from build123d import *

# Parameters (mm, degrees)
SKETCH1_W           = 42
SKETCH1_H           = 42
SKETCH1_R           = 1.9
BOSS_EXTRUDE1_DEPTH = 10
SKETCH2_W           = 12
SKETCH2_H           = 150
BOSS_EXTRUDE2_DEPTH = 10
SKETCH3_W           = 12
SKETCH3_H           = 3.75
BOSS_EXTRUDE3_DEPTH = 12
CHAMFER1_SIZE       = 3.75
CHAMFER1_SIZE_2     = 12.265697319
SKETCH4_R           = 1.375
CUT_EXTRUDE1_DEPTH  = 12
SKETCH5_W           = 42
SKETCH5_H           = 42
SKETCH5_R           = 1.65
SKETCH5_R_2         = 5
BOSS_EXTRUDE4_DEPTH = 7.5
SKETCH6_R           = 12.5
CUT_EXTRUDE2_DEPTH  = 5.2
FILLET1_R           = 4
FILLET2_R           = 9
SKETCH8_R           = 3.5
CUT_EXTRUDE4_DEPTH  = 1.2
BOSS_EXTRUDE7_DEPTH = 6


with BuildPart() as part:
    # Sketch1 → Boss-Extrude1 (new body)
    with BuildSketch(Plane(origin=(0, 0, 0), x_dir=(0, 0, -1), z_dir=(1, 0, 0))):
        Rectangle(SKETCH1_W, SKETCH1_H)
        with Locations((16, -16)):
            Circle(SKETCH1_R, mode=Mode.SUBTRACT)
        with Locations((-16, -16)):
            Circle(SKETCH1_R, mode=Mode.SUBTRACT)
        with Locations((-16, 16)):
            Circle(SKETCH1_R, mode=Mode.SUBTRACT)
        with Locations((16, 16)):
            Circle(SKETCH1_R, mode=Mode.SUBTRACT)
    extrude(amount=BOSS_EXTRUDE1_DEPTH)

    # Sketch2 → Boss-Extrude2 (add)
    with BuildSketch(Plane.ZY):
        with Locations((0, -29)):
            Rectangle(SKETCH2_W, SKETCH2_H)
    extrude(amount=-BOSS_EXTRUDE2_DEPTH)

    # Sketch3 → Boss-Extrude3 (add)
    with BuildSketch(Plane.ZY):
        with Locations((0, 40.375)):
            Rectangle(SKETCH3_W, SKETCH3_H)
        with Locations((0, -64.575)):
            Rectangle(SKETCH3_W, SKETCH3_H)
    extrude(amount=BOSS_EXTRUDE3_DEPTH)

    # Chamfer1
    # the kernel refuses this chamfer: 12.265697319, 3.75 mm, written as the material it adds along each edge
    with BuildSketch(Plane(origin=(0, 42.25, -6), x_dir=(0.11964200288050787, 0.9928170985366542, 0), z_dir=(0, 0, 1))) as chamfer1_piece_1_section:
        Polygon((CHAMFER1_SIZE * 0.992817098537, CHAMFER1_SIZE * 0.119642002881), (-CHAMFER1_SIZE_2 * 0.119642002884, CHAMFER1_SIZE_2 * 0.992817098562), (0, 0), align=None)
    chamfer1_piece_1 = extrude(amount=12, mode=Mode.PRIVATE)
    chamfer1_piece_1 = split(chamfer1_piece_1, bisect_by=Plane(origin=(-4.172539525, 46, 0), z_dir=(0, -1, 0)), keep=Keep.TOP, mode=Mode.PRIVATE)
    chamfer1_piece_1 = split(chamfer1_piece_1, bisect_by=Plane(origin=(-12, 43.383581674, 0), z_dir=(1, 0, 0)), keep=Keep.TOP, mode=Mode.PRIVATE)
    add(chamfer1_piece_1)
    with BuildSketch(Plane(origin=(0, -66.45, -6), x_dir=(0.11964200288050787, -0.9928170985366542, 0), z_dir=(0, 0, 1))) as chamfer1_piece_2_section:
        Polygon((CHAMFER1_SIZE * 0.992817098537, -CHAMFER1_SIZE * 0.119642002881), (-CHAMFER1_SIZE_2 * 0.119642002884, -CHAMFER1_SIZE_2 * 0.992817098562), (0, 0), align=None)
    chamfer1_piece_2 = extrude(amount=12, mode=Mode.PRIVATE)
    chamfer1_piece_2 = split(chamfer1_piece_2, bisect_by=Plane(origin=(-12, -67.58994207, 0), z_dir=(1, 0, 0)), keep=Keep.TOP, mode=Mode.PRIVATE)
    add(chamfer1_piece_2)

    # Sketch4 → Cut-Extrude1 (cut)
    with BuildSketch(Plane.ZY):
        with Locations((0, 25.4)):
            Circle(SKETCH4_R)
        with Locations((0, 0.4)):
            Circle(SKETCH4_R)
        with Locations((0, -24.6)):
            Circle(SKETCH4_R)
        with Locations((0, -49.6)):
            Circle(SKETCH4_R)
    extrude(amount=-CUT_EXTRUDE1_DEPTH, mode=Mode.SUBTRACT)

    # Sketch5 → Boss-Extrude4 (add)
    # profile 1 of 2: a face of its own
    with BuildSketch(Plane.XZ.offset(104)):
        Polygon((10, -56), (10, 6), (0, 6), (-34.5, -14), (7.5, -14), (7.5, -56), align=None)
    # profile 2 of 2: a face of its own
    with BuildSketch(Plane.XZ.offset(104)):
        with Locations((-13.5, -35)):
            Rectangle(SKETCH5_W, SKETCH5_H)
        with Locations(Location((-29, -50.5, 0), (0, 0, 270))):
            Circle(SKETCH5_R, mode=Mode.SUBTRACT)
        with Locations(Location((-13.5, -35, 0), (0, 0, 270))):
            Circle(SKETCH5_R_2, mode=Mode.SUBTRACT)
        with Locations(Location((2, -50.5, 0), (0, 0, 270))):
            Circle(SKETCH5_R, mode=Mode.SUBTRACT)
        with Locations(Location((-29, -19.5, 0), (0, 0, 270))):
            Circle(SKETCH5_R, mode=Mode.SUBTRACT)
        with Locations(Location((2, -19.5, 0), (0, 0, 270))):
            Circle(SKETCH5_R, mode=Mode.SUBTRACT)
    extrude(amount=BOSS_EXTRUDE4_DEPTH)

    # Sketch6 → Cut-Extrude2 (cut)
    with BuildSketch(Plane.XZ.offset(111.5)):
        with Locations(Location((-13.5, -35, 0), (0, 0, 270))):
            Circle(SKETCH6_R)
    extrude(amount=-CUT_EXTRUDE2_DEPTH, mode=Mode.SUBTRACT)

    # Fillet1
    fillet1_edges = [part.edges().sort_by_distance(p)[0] for p in [
        (-34.5, -107.75, -56),
        (10, -107.75, -56),
        (-34.5, -107.75, -14),
        (5, -21, 6),
        (5, -21, -6),
        (5, 21, -6),
        (5, 21, 6),
        (5, -21, -21),
        (5, -21, 21),
        (5, 21, 21),
        (5, 21, -21),
    ]]
    fillet(fillet1_edges, radius=FILLET1_R)

    # Fillet2
    fillet2_edges = [part.edges().sort_by_distance(p)[0] for p in [
        (5, -104, -6),
        (0, -104, 0),
    ]]
    fillet(fillet2_edges, radius=FILLET2_R)

    # Sketch8 → Cut-Extrude4 (cut)
    with BuildSketch(Plane(origin=(0, -104, 0), x_dir=(1, 0, 0), z_dir=(0, 1, 0))):
        with Locations(Location((-29, 50.5, 0), (0, 0, 270))):
            Circle(SKETCH8_R)
        with Locations(Location((2, 50.5, 0), (0, 0, 270))):
            Circle(SKETCH8_R)
        with Locations(Location((2, 19.5, 0), (0, 0, 270))):
            Circle(SKETCH8_R)
        with Locations(Location((-29, 19.5, 0), (0, 0, 270))):
            Circle(SKETCH8_R)
    extrude(amount=-CUT_EXTRUDE4_DEPTH, mode=Mode.SUBTRACT)

    # Sketch11 → Boss-Extrude7 (add)
    with BuildSketch(Plane.XZ.offset(111.5)):
        Polygon((8.3, 6), (10, 6), (10, 9.2), (2.9, 9.2), (2.9, 7.5), (3.9, 7.5), (8.3, 7.5), align=None)
        Polygon((3.9, 7.5), (2.9, 7.5), (3.433368825, 6.8), align=None)
    extrude(amount=-BOSS_EXTRUDE7_DEPTH)


solid = part.part
Work out the finished part from the listing and answer in its coordinate system (mm). A direction names the side the tool comes from. Give positions to 0.01 mm unless a question says otherwise; leave off trailing zeros. Order: outer loops, then holes, each group sorted by start corner. A loop starts at its lowest first (then second) coordinate and runs counter-clockwise, first axis right, second up. Notation, with made-up numbers: (-9.75, -16.75) -> (29.25, -16.75) arc R32 cw to (29.25, 21.25) -> close; hole circle Ø9 at (2.5, 21.5). An arc over 180 degrees is marked (long way). Answer as a JSON object with one key per item and string values. Group by question number.
1. The mould has two halves that part along X. Classify faces 5 (the flat face through (-6, 38.5, 0)), 6 (the cylindrical face through (-12.95, -108.936, -22.512)), 7 (the cylindrical face through (-33.98, -107.8, -14.33)), 8 (the flat face through (-31, -105.2, -19)): released by +X, released by -X, zero draft, split by the parting line, or undercut.
2. Section C-C on x = -13.5 is taken. Determine the outline of the cut face in (y, z).
3. Section D-D on z = -19.5 is taken. Determine the outline of the cut face in (x, y).
4. Consider line 1 along Y through (x, z) = (5.75, -16); line 2 along X through (y, z) = (-104.5, -19.5); line 3 along X through (y, z) = (-109, -50.5). Determine where each line is inside the solid, lowest interval first. Write a range as [from, to].
5. A tool of negligible diameter and unlimited length cuts with its end or side. For faces 1 (the flat face through (5, 21, 14)), 2 (the cylindrical face through (3.05, -104.59, -16.16)), 3 (the flat face through (5, -21, 14)), 4 (the flat face through (-16.026, -106.801, -3.29)), from which of +Z, -Z, +X, -X, +Y, -Y can it reach the whole face along a straight path? Write none if from no direction.
6. Section A-A on z = -35 is taken. Determine the outline of the cut face in (x, y), plus the area to 3 significant figures.
7. Flat-ended cylindrical pins translate along their axes: pin 1 Ø1 at (x, z) = (6, 7) entering from +Y; pin 2 Ø3.5 at (x, z) = (5, 13.5) entering from -Y; pin 3 Ø6 at (x, z) = (-27, -43) entering from +Y. Find the tip coordinate at first contact, or state that the pin passes through.
8. Section B-B on x = -29 is taken. Determine the outline of the cut face in (y, z), plus the area to 3 significant figures.
Result sheet:
{
 "1": {"face 5": "zero draft", "face 6": "undercut", "face 7": "released by -X", "face 8": "undercut"},
 "2": {"outline": "(-111.5, -56) -> (-104, -56) -> (-104, -40) -> (-106.3, -40) -> (-106.3, -47.5) -> (-111.5, -47.5) -> close; (-111.5, -22.5) -> (-106.3, -22.5) -> (-106.3, -30) -> (-104, -30) -> (-104, -1.83) -> (-111.5, -1.83) -> close"},
 "3": {"outline": "(-34.5, -111.5) -> (-30.65, -111.5) -> (-30.65, -105.2) -> (-32.5, -105.2) -> (-32.5, -104) -> (-34.5, -104) -> close; (-27.35, -111.5) -> (0.35, -111.5) -> (0.35, -105.2) -> (-1.5, -105.2) -> (-1.5, -104) -> (-25.5, -104) -> (-25.5, -105.2) -> (-27.35, -105.2) -> close; (0, -20.12) -> (10, -20.12) -> (10, 20.12) -> (0, 20.12) -> close; (3.65, -111.5) -> (10, -111.5) -> (10, -104) -> (5.5, -104) -> (5.5, -105.2) -> (3.65, -105.2) -> close"},
 "4": {"line 1": "y = [-111.5, -104], [-21, -17.9], [-14.1, 14.1], [17.9, 21]", "line 2": "x = [-34.5, -32.5], [-25.5, -1.5], [5.5, 10]", "line 3": "x = [-34.5, -30.65], [-27.35, 0.35], [3.65, 10]"},
 "5": {"face 1": "+Z, +X, -X, +Y", "face 2": "none", "face 3": "+Z, +X, -X, -Y", "face 4": "+Z, -X, -Y"},
 "6": {"outline": "(-34.5, -111.5) -> (-26, -111.5) -> (-26, -106.3) -> (-18.5, -106.3) -> (-18.5, -104) -> (-34.5, -104) -> close; (-8.5, -106.3) -> (-1, -106.3) -> (-1, -111.5) -> (10, -111.5) -> (10, -104) -> (-8.5, -104) -> close", "area": "181 mm^2"},
 "7": {"pin 1": "stops at y = 23.06", "pin 2": "stops at y = -21", "pin 3": "stops at y = -104"},
 "8": {"outline": "(-111.5, -56) -> (-104, -56) -> (-104, -54) -> (-105.2, -54) -> (-105.2, -52.15) -> (-111.5, -52.15) -> close; (-111.5, -48.85) -> (-105.2, -48.85) -> (-105.2, -47) -> (-104, -47) -> (-104, -23) -> (-105.2, -23) -> (-105.2, -21.15) -> (-111.5, -21.15) -> close; (-111.5, -17.85) -> (-105.2, -17.85) -> (-105.2, -16) -> (-104, -16) -> (-104, -10.81) -> (-111.5, -10.81) -> close", "area": "281 mm^2"}
}
